```python
from build123d import *

# Parameters (mm, degrees)
ESQUISSE1_W             = 10
ESQUISSE1_H             = 20
BOSS_EXTRU_1_DEPTH      = 11
BOSS_EXTRU_1_2_DEPTH    = 11
ESQUISSE3_W             = 40
ESQUISSE3_H             = 20
BOSS_EXTRU_2_DEPTH      = 12
ESQUISSE4_R             = 3.2
ENL_V_MAT_EXTRU_1_DEPTH = 12
ESQUISSE1_3_R           = 2
ENL_V_MAT_EXTRU_3_DEPTH = 15
CHANFREIN1_SIZE         = 3
CONG_1_R                = 3
ESQUISSE6_W             = 10.5
ESQUISSE6_H             = 20
ENL_V_MAT_EXTRU_5_DEPTH = 5


with BuildPart() as part:
    # Esquisse1 → Boss.-Extru.1 (new body)
    with BuildSketch(Plane(origin=(0, 0, 0), x_dir=(1, 0, 0), z_dir=(0, 1, 0))):
        with Locations((-15, 0)):
            Rectangle(ESQUISSE1_W, ESQUISSE1_H)
    extrude(amount=BOSS_EXTRU_1_DEPTH)



with BuildPart() as body_2:
    # Esquisse1 → Boss.-Extru.1 2 (new body)
    with BuildSketch(Plane(origin=(0, 0, 0), x_dir=(1, 0, 0), z_dir=(0, 1, 0))):
        with Locations((15, 0)):
            Rectangle(ESQUISSE1_W, ESQUISSE1_H)
    extrude(amount=BOSS_EXTRU_1_2_DEPTH)


with BuildPart() as part_1:
    add(part.part)

    add(body_2.part)  # Boss.-Extru.2 merges body 2
    # Esquisse3 → Boss.-Extru.2 (add)
    with BuildSketch(Plane(origin=(0, 11, 0), x_dir=(1, 0, 0), z_dir=(0, 1, 0))):
        Rectangle(ESQUISSE3_W, ESQUISSE3_H)
    extrude(amount=BOSS_EXTRU_2_DEPTH)

    # Esquisse4 → Enl_v. mat.-Extru.1 (cut)
    with BuildSketch(Plane(origin=(0, 23, 0), x_dir=(1, 0, 0), z_dir=(0, 1, 0))):
        Circle(ESQUISSE4_R)
    extrude(amount=-ENL_V_MAT_EXTRU_1_DEPTH, mode=Mode.SUBTRACT)

    # Esquisse1_3 → Enl_v. mat.-Extru.3 (cut)
    with BuildSketch(Plane(origin=(0, 0, 0), x_dir=(1, 0, 0), z_dir=(0, 1, 0))):
        with Locations((-15, 0)):
            Circle(ESQUISSE1_3_R)
        with Locations((15, 0)):
            Circle(ESQUISSE1_3_R)
    extrude(amount=ENL_V_MAT_EXTRU_3_DEPTH, mode=Mode.SUBTRACT)

    # Chanfrein1
    chanfrein1_edges = [part_1.edges().sort_by_distance(p)[0] for p in [
        (20, 11.5, 10),
        (20, 11.5, -10),
        (10, 5.5, -10),
        (10, 5.5, 10),
        (-20, 11.5, 10),
        (-20, 11.5, -10),
        (-10, 5.5, -10),
        (-10, 5.5, 10),
    ]]
    chamfer(chanfrein1_edges, length=CHANFREIN1_SIZE)

    # Cong_1
    cong_1_edges = [part_1.edges().sort_by_distance(p)[0] for p in [
        (10, 5.5, 7),
        (10, 5.5, -7),
        (-17, 11.5, -10),
        (-13, 5.5, -10),
        (17, 11.5, -10),
        (13, 5.5, -10),
        (20, 11.5, 7),
        (20, 11.5, -7),
        (-17, 11.5, 10),
        (17, 11.5, 10),
        (-13, 5.5, 10),
        (13, 5.5, 10),
        (-10, 5.5, 7),
        (-10, 5.5, -7),
        (-20, 11.5, 7),
        (-20, 11.5, -7),
    ]]
    fillet(cong_1_edges, radius=CONG_1_R)

    # Esquisse6 → Enl_v. mat.-Extru.5 (cut)
    with BuildSketch(Plane(origin=(0, 14.5, 0), x_dir=(-1, 0, 0), z_dir=(0, -1, 0))):
        Rectangle(ESQUISSE6_W, ESQUISSE6_H)
    extrude(amount=-ENL_V_MAT_EXTRU_5_DEPTH, mode=Mode.SUBTRACT)


solid = part_1.part
```
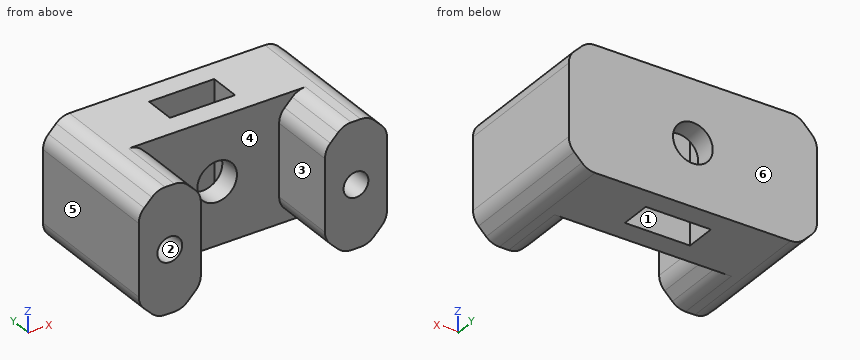
The listing builds one solid part. Answer for the finished solid, in the listing's coordinates (mm). Face numbers are marked on the shaded views. A direction names the side the tool comes from. Round coordinates to 2 decimals unless told otherwise and drop trailing zeros. Order: outer loops, then holes, each group sorted by start corner. A loop starts at its lowest first (then second) coordinate and runs counter-clockwise, first axis right, second up. Notation, with made-up numbers: (-29.75, -18.75) - (-0.75, -18.75) arc R16 ccw to (-0.75, -3.75) - close; hole circle Ø7 at (-27.75, 75). An arc over 180 degrees is marked (long way). Put each result on its own line as item: value. Start each with the question number.
(1) Find section B-B (y = 5). State how many separate pieces and enclosed holes the cut face has, plus the area to 3 significant figures.
(2) Find section A-A (z = 0). Give the vertices of the cut face in (x, y), plus the area to 3 significant figures.
(3) Find section D-D (x = -15). Give the vertices of the cut face in (y, z).
(4) Determine the mould class of the marked faces 4, 5 and 6 for opening direction X: released by +X, released by -X, zero draft, split by the parting line, or undercut.
(5) Find section C-C (x = 0). Give the vertices of the cut face in (y, z).
(6) Straight lines are drawn through the part: probe 1 along X at (y, z) = (12.25, 0); probe 2 along X at (y, z) = (3.25, 0); probe 3 along X at (y, z) = (16.5, -4.25). For each, find the intervals that lie inside material, in ascending order. Write a range as from..to.
(7) For the marked faces 1, 2 and 3, determine the directions among +Z, -Z, +X, -X, +Y, -Y from which every point of the face is accessible in a straight line to the end or side of a thin tool.
(8) Given P1, Ø3, axis at x = 1, z = -2.5, coming from the -Y side; P2, Ø4, axis at x = 0, z = 0, coming from the -Y side; P3, Ø1.2, axis at x = -15, z = -0.5, coming from the -Y side, each flat-ended and moving along its own axis, determine where each tip first touches the part or whether it passes through.
Reply:
1. separate pieces: 2
1. enclosed holes: 2
1. area: 336 mm^2
2. outline: (-20, 0) - (-17, 0) - (-17, 15) - (-13, 15) - (-13, 0) - (-10, 0) - (-10, 11) - (-3.2, 11) - (-3.2, 14.5) - (-5.25, 14.5) - (-5.25, 19.5) - (-3.2, 19.5) - (-3.2, 23) - (-20, 23) - close; (3.2, 11) - (10, 11) - (10, 0) - (13, 0) - (13, 15) - (17, 15) - (17, 0) - (20, 0) - (20, 23) - (3.2, 23) - (3.2, 19.5) - (5.25, 19.5) - (5.25, 14.5) - (3.2, 14.5) - close
2. area: 483 mm^2
3. outline: (0, -10) - (23, -10) - (23, 10) - (0, 10) - (0, 2) - (15, 2) - (15, -2) - (0, -2) - close
4. face 4: undercut
4. face 5: released by -X
4. face 6: zero draft
5. outline: (11, -10) - (14.5, -10) - (14.5, -3.2) - (11, -3.2) - close; (11, 3.2) - (14.5, 3.2) - (14.5, 10) - (11, 10) - close; (19.5, -10) - (23, -10) - (23, -3.2) - (19.5, -3.2) - close; (19.5, 3.2) - (23, 3.2) - (23, 10) - (19.5, 10) - close
6. probe 1: -20..-17, -13..-3.2, 3.2..13, 17..20
6. probe 2: -20..-17, -13..-10, 10..13, 17..20
6. probe 3: -20..-5.25, 5.25..20
7. face 1: +Z, -Z
7. face 2: -Y
7. face 3: +Z, -Z, -Y
8. P1: y = 11
8. P2: through
8. P3: y = 15
